```python
from build123d import *

# Parameters (mm, degrees)
SKETCH_1_W          = 220
SKETCH_1_H          = 114
SKETCH_1_R          = 2.5
SKETCH_1_R_2        = 3
SKETCH_1_R_3        = 5
SKETCH_1_R_4        = 2
SKETCH_1_R_5        = 3.5
SKETCH_1_W_2        = 135
SKETCH_1_H_2        = 8
SKETCH_1_W_3        = 53.5
SKETCH_1_W_4        = 33
EXTRUDE_1_DEPTH     = 1.5
SKETCH_2_W          = 55
SKETCH_2_H          = 14.5
CUT_EXTRUDE_1_DEPTH = 248.800322841
FILLET_1_R          = 5
SKETCH_3_W          = 19
SKETCH_3_H          = 114
CUT_EXTRUDE_2_DEPTH = 248.800322841
FILLET_2_R          = 6


with BuildPart() as part:
    # 草图1 → 凸台-拉伸1 (new, symmetric)
    with BuildSketch(Plane(origin=(0, 0, 0), x_dir=(1, 0, 0), z_dir=(0, 1, 0))):
        with Locations((-110, 57)):
            Rectangle(SKETCH_1_W, SKETCH_1_H)
        with Locations(Location((-71, 102.5, 0), (0, 0, 270))):
            Circle(SKETCH_1_R, mode=Mode.SUBTRACT)
        with Locations(Location((-109, 102.5, 0), (0, 0, 270))):
            Circle(SKETCH_1_R, mode=Mode.SUBTRACT)
        with Locations(Location((-141.312887166, 80.5, 0), (0, 0, 270))):
            Circle(SKETCH_1_R, mode=Mode.SUBTRACT)
        with Locations(Location((-109.312887166, 80.5, 0), (0, 0, 270))):
            Circle(SKETCH_1_R, mode=Mode.SUBTRACT)
        with Locations(Location((-109, 10.5, 0), (0, 0, 270))):
            Circle(SKETCH_1_R, mode=Mode.SUBTRACT)
        with Locations(Location((-71, 10.5, 0), (0, 0, 270))):
            Circle(SKETCH_1_R, mode=Mode.SUBTRACT)
        with Locations(Location((-76, 47, 0), (0, 0, 270))):
            Circle(SKETCH_1_R_2, mode=Mode.SUBTRACT)
        with Locations(Location((-76, 83, 0), (0, 0, 270))):
            Circle(SKETCH_1_R_2, mode=Mode.SUBTRACT)
        with Locations(Location((-170, 65, 0), (0, 0, 270))):
            Circle(SKETCH_1_R_2, mode=Mode.SUBTRACT)
        with Locations(Location((-170.312887166, 21.5, 0), (0, 0, 270))):
            Circle(SKETCH_1_R_3, mode=Mode.SUBTRACT)
        with Locations(Location((-181.312887166, 21.5, 0), (0, 0, 270))):
            Circle(SKETCH_1_R, mode=Mode.SUBTRACT)
        with Locations(Location((-210.002887166, 37.50000026, 0), (0, 0, 270))):
            Circle(SKETCH_1_R_4, mode=Mode.SUBTRACT)
        with Locations(Location((-210.002887166, 5.5, 0), (0, 0, 270))):
            Circle(SKETCH_1_R_4, mode=Mode.SUBTRACT)
        with Locations(Location((-210.002887166, 21.5, 0), (0, 0, 270))):
            Circle(SKETCH_1_R_5, mode=Mode.SUBTRACT)
        with BuildLine():
            Line((-193.157887166, 18.743662964), (-193.157887166, 11.743662964))
            ThreePointArc((-193.157887166, 11.743662964), (-193.836926328, 9.268099132), (-195.683983559, 7.485435381))
            ThreePointArc((-195.683983559, 7.485435381), (-196.460455274, 4.734904062), (-193.694496162, 4.015320115))
            ThreePointArc((-193.694496162, 4.015320115), (-190.370630742, 7.428094707), (-189.157887166, 12.035085564))
            Line((-189.157887166, 12.035085564), (-189.157887166, 18.743662964))
            ThreePointArc((-189.157887166, 18.743662964), (-191.157887166, 20.743662964), (-193.157887166, 18.743662964))
        make_face(mode=Mode.SUBTRACT)
        with Locations((-89.5, 22.5)):
            Rectangle(SKETCH_1_W_2, SKETCH_1_H_2, mode=Mode.SUBTRACT)
        with Locations((-165.25, 32.5)):
            Rectangle(SKETCH_1_W_3, SKETCH_1_H_2, mode=Mode.SUBTRACT)
        with Locations((-125.5, 91.5)):
            Rectangle(SKETCH_1_W_4, SKETCH_1_H_2, mode=Mode.SUBTRACT)
        with BuildLine():
            ThreePointArc((-196.226976492, 65.454109411), (-198.733501828, 64.143639747), (-197.423032164, 61.637114411))
            ThreePointArc((-197.423032164, 61.637114411), (-187.463332326, 57.014316596), (-179.039469146, 49.971276796))
            ThreePointArc((-179.039469146, 49.971276796), (-176.213519698, 49.852914148), (-176.09515705, 52.678863596))
            ThreePointArc((-176.09515705, 52.678863596), (-185.320120262, 60.391688659), (-196.226976492, 65.454109411))
        make_face(mode=Mode.SUBTRACT)
    extrude(amount=EXTRUDE_1_DEPTH, both=True)

    # 草图2 → 切除-拉伸1 (cut, through all)
    with BuildSketch(Plane(origin=(0, 1.5, 0), x_dir=(1, 0, 0), z_dir=(0, 1, 0))):
        with Locations((-158.812887166, 7.25)):
            Rectangle(SKETCH_2_W, SKETCH_2_H)
    extrude(amount=-CUT_EXTRUDE_1_DEPTH, mode=Mode.SUBTRACT)

    # 圆角1
    fillet_1_edges = [part.edges().sort_by_distance(p)[0] for p in [
        (-186.312887166, 0, 0),
        (-186.312887166, 0, -14.5),
        (-131.312887166, 0, -14.5),
        (-131.312887166, 0, 0),
    ]]
    fillet(fillet_1_edges, radius=FILLET_1_R)

    # 草图3 → 切除-拉伸2 (cut, through all)
    with BuildSketch(Plane(origin=(0, 1.5, 0), x_dir=(1, 0, 0), z_dir=(0, 1, 0))):
        Polygon((-220, 54), (-150, 114), (-220, 114), align=None)
        with Locations((-9.5, 57)):
            Rectangle(SKETCH_3_W, SKETCH_3_H)
    extrude(amount=-CUT_EXTRUDE_2_DEPTH, mode=Mode.SUBTRACT)

    # 圆角2
    fillet_2_edges = [part.edges().sort_by_distance(p)[0] for p in [
        (-220, 0, -54),
        (-150, 0, -114),
        (-19, 0, 0),
        (-19, 0, -114),
        (-220, 0, 0),
    ]]
    fillet(fillet_2_edges, radius=FILLET_2_R)


solid = part.part
```
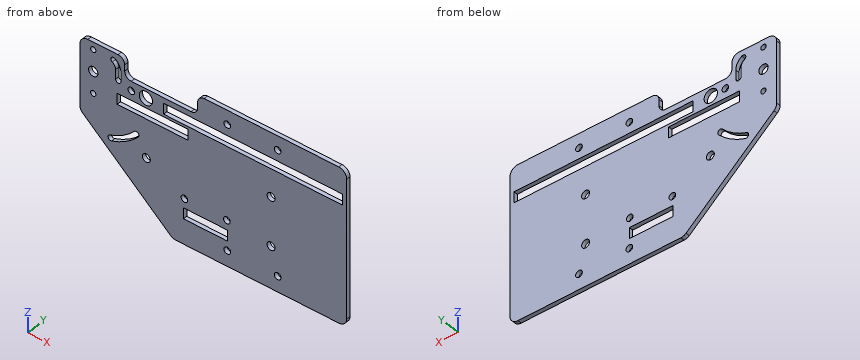
Source: CAD feature listing. Evaluate the final solid. Frame: model axes, mm. Give positions to 0.01 mm unless a question says otherwise; leave off trailing zeros. Order: outer loops, then holes, each group sorted by start corner. A loop starts at its lowest first (then second) coordinate and runs counter-clockwise, first axis right, second up.
(1) Section query A-A (x = -45.5). Return the cut outline in (y, z).
(2) Material intervals for line 1 along Z through (x, y) = (-114, -0.5); line 2 along Z through (x, y) = (-145, -0.35); line 3 along X through (y, z) = (0.8, -21.5), sorted ascending.
(3) Section query B-B (x = -71). Return the cut outline in (y, z), plus the area to 3 significant figures.
(4) Contact query for a flat-ended pin moving along its axis: P1, Ø0.9, axis at x = -156.5, y = -0.5, coming from the +Z side. Output: stop coordinate, or through.
(5) Section query D-D (z = -102.5). Return the cut outline in (x, y).
(6) Section query C-C (z = -90). Return the cut outline in (x, y), plus the area to 3 significant figures.
Outcome:
1. outline: (-1.5, -114) - (1.5, -114) - (1.5, -26.5) - (-1.5, -26.5) - close; (-1.5, -18.5) - (1.5, -18.5) - (1.5, 0) - (-1.5, 0) - close
2. line 1: z = -114 to -95.5, -87.5 to -26.5, -18.5 to 0
2. line 2: z = -114 to -36.5, -28.5 to -26.5, -18.5 to -14.5
2. line 3: x = -220 to -213.5, -206.5 to -183.81, -178.81 to -175.31, -165.31 to -157, -22 to -19
3. outline: (-1.5, -114) - (1.5, -114) - (1.5, -105) - (-1.5, -105) - close; (-1.5, -100) - (1.5, -100) - (1.5, -26.5) - (-1.5, -26.5) - close; (-1.5, -18.5) - (1.5, -18.5) - (1.5, -13) - (-1.5, -13) - close; (-1.5, -8) - (1.5, -8) - (1.5, 0) - (-1.5, 0) - close
3. area: 288 mm2
4. P1: stops at z = -14.5
5. outline: (-163.42, -1.5) - (-111.5, -1.5) - (-111.5, 1.5) - (-163.42, 1.5) - close; (-106.5, -1.5) - (-73.5, -1.5) - (-73.5, 1.5) - (-106.5, 1.5) - close; (-68.5, -1.5) - (-19, -1.5) - (-19, 1.5) - (-68.5, 1.5) - close
6. outline: (-178, -1.5) - (-142, -1.5) - (-142, 1.5) - (-178, 1.5) - close; (-109, -1.5) - (-19, -1.5) - (-19, 1.5) - (-109, 1.5) - close
6. area: 378 mm2
